```python
from build123d import *

# Parameters (mm, degrees)
SKETCH1_W          = 6
SKETCH1_H          = 1.5
CHAMFER1_SIZE      = 0.375
CUT_EXTRUDE2_DEPTH = 1.155


with BuildPart() as part:
    # Sketch1 → Revolve1 (revolve)
    with BuildSketch(Plane(origin=(0, 0, 0), x_dir=(0, 0, -1), z_dir=(1, 0, 0))):
        with Locations((4.65, 0.75)):
            Rectangle(SKETCH1_W, SKETCH1_H)
    revolve(axis=Axis((0, 0, -7.65), (0, 0, 1)))

    # Chamfer1
    chamfer1_edges = [part.edges().sort_by_distance(p)[0] for p in [
        (0, -1.5, -7.65),
    ]]
    chamfer(chamfer1_edges, length=CHAMFER1_SIZE)

    # Sketch7 → Revolve2 (revolve)
    with BuildSketch(Plane(origin=(0, 0, 0), x_dir=(0, 0, -1), z_dir=(1, 0, 0)), mode=Mode.PRIVATE) as revolve2_sk:
        with BuildLine():
            Line((1.4025, 2.85), (1.65, 2.85))
            Line((1.65, 2.85), (1.65, 0))
            Line((1.65, 0), (0, 0))
            Line((0, 0), (0, 1.5))
            ThreePointArc((0, 1.5), (0.59512511, 2.285251969), (1.4025, 2.85))
        make_face()
    revolve(revolve2_sk.sketch.rotate(Axis((0, 0, 0), (0, 0, -1)), 180), axis=Axis((0, 0, 0), (0, 0, -1)))

    # Sketch5 → Cut-Extrude2 (cut)
    with BuildSketch(Plane.XY):
        Polygon((1, -0.577350269), (1, 0.577350269), (0, 1.154700538), (-1, 0.577350269), (-1, -0.577350269), (0, -1.154700538), align=None)
    extrude(amount=-CUT_EXTRUDE2_DEPTH, mode=Mode.SUBTRACT)

    # Cut-Extrude3 cone 1 section (on through the dimple's axis) → Cut-Extrude3 (revolve, cut)
    with BuildSketch(Plane(origin=(0, 0, 0), x_dir=(0, -1, 0), z_dir=(1, 0, 0))):
        Polygon((0, 0), (1.154700538, 0), (0, 1.154700538), align=None)
    revolve(axis=Axis((0, 0, 0), (0, 0, -1)), mode=Mode.SUBTRACT)


solid = part.part
```
For this review, take the finished solid that the model builds, in its own axes (mm). A direction names the side the tool comes from. Round coordinates to 2 decimals unless told otherwise and drop trailing zeros. Loops run counter-clockwise (first coordinate to the right, second up) from the corner with the lowest first, then second, coordinate; pieces in that order, holes last.
(1) We need section D-D (z = -1.25). Give the boundary of the cut face in (x, y).
Returned:
outline: circle Ø5.54 at (0, 0)
(2) We need section C-C (x = 2.05). Give the boundary of the cut face in (y, z), plus the area to 3 significant figures.
Returned:
outline: (-1.98, -1.65) - (1.98, -1.65) - (1.98, -1.4) arc R2.42 ccw to (-1.98, -1.4) - close
area: 3.84 mm2
(3) Wall thickness on line 1 along Y through (x, z) = (0, -5); line 2 along Y through (x, z) = (-0.7, -0.5); line 3 along Z through (x, y) = (0, -0.45) (3 decimals): over which ranges is each line inside the solid? List them lowest first.
Returned:
line 1: y = -1.5 to 1.5
line 2: y = -2.07 to -0.75, 0.75 to 2.07
line 3: z = -7.65 to -1.155
(4) We need section B-B (z = -5.75). Give the boundary of the cut face in (x, y), plus the area to 3 significant figures.
Returned:
outline: circle Ø3 at (0, 0)
area: 7.07 mm2
(5) Tool access review of faces 1 (the flat face through (0.51, 0.86, -0.57)), 2 (the flat face through (0, 0, -7.65)): name each direction out of +Z, -Z, +X, -X, +Y, -Y from which nothing blocks a thin tool from reaching the whole face with its end or side.
Returned:
face 1: +Z
face 2: -Z, +X, -X, +Y, -Y
(6) Mouldability with a two-part tool opening along Y and no side actions: class faces 3 (the flat face through (-0.49, 0.87, -0.57)), 4 (the cylindrical face through (-0.07, -1.5, -4.5)), 5 (the flat face through (1.2, -1.2, -1.65)) as released by +Y, released by -Y, zero draft, split by the parting line, or undercut.
Returned:
face 3: undercut
face 4: split by the parting line
face 5: zero draft
(7) Clearance check with flat-ended pins moving along their axes: P1, Ø0.9, axis at y = 0, z = -0.5, coming from the -X side; P2, Ø3, axis at x = 0.5, z = -5.5, coming from the -Y side; P3, Ø1, axis at x = -2, y = 1.5, coming from the +Z side. State where each tip first meets the part, or that it passes through.
Returned:
P1: stops at x = -2.58
P2: stops at y = -1.5
P3: stops at z = -0.33
